Source: CAD feature listing. Evaluate the final solid. Frame: model axes, mm. A direction names the side the tool comes from. Give positions to 0.01 mm unless a question says otherwise; leave off trailing zeros. Order: outer loops, then holes, each group sorted by start corner. A loop starts at its lowest first (then second) coordinate and runs counter-clockwise, first axis right, second up.
```python
from build123d import *

# Parameters (mm, degrees)
SKETCH_1_W               = 994
SKETCH_1_H               = 740
EXTRUDE_1_DEPTH          = 4
CUT_EXTRUDE_3_DEPTH      = 1240.214267187
SKETCH_10_W              = 20
SKETCH_10_H              = 20
SKETCH_10_W_2            = 40
SKETCH_10_H_2            = 40
SKETCH_10_W_3            = 30
SKETCH_10_H_3            = 30
CUT_EXTRUDE_4_DEPTH      = 1240.214267187
SKETCH_11_W              = 11
SKETCH_11_H              = 15.8
CUT_EXTRUDE_5_DEPTH      = 1240.214267187
SKETCH_2_R               = 2.6
CUT_EXTRUDE_1_DEPTH      = 1240.214267187
SKETCH_12_W              = 8
SKETCH_12_H              = 20
CUT_EXTRUDE_6_DEPTH      = 1240.214267187
CUT_EXTRUDE_7_DEPTH      = 1240.214267187
CUT_EXTRUDE_7_DEPTH_BACK = 1240.214267187
SKETCH_13_W              = 4.2
SKETCH_13_H              = 20.2
SKETCH_6_W               = 26.45
SKETCH_6_H               = 740
EXTRUDE_2_DEPTH          = 4
SKETCH_8_W               = 5.8
SKETCH_8_H               = 10.5
CUT_EXTRUDE_2_DEPTH      = 1243.700125734
SKETCH_14_R              = 2.6
CUT_EXTRUDE_8_DEPTH      = 1243.700125734
FILLET_1_R               = 1.5
FILLET_2_R               = 5.5
FILLET_4_R               = 2.5


with BuildPart() as part:
    # Эскиз1 → Бобышка-Вытянуть1 (new body)
    with BuildSketch(Plane.XY):
        with Locations((497, 370)):
            Rectangle(SKETCH_1_W, SKETCH_1_H)
    extrude(amount=EXTRUDE_1_DEPTH)

    # Эскиз9 → Вырез-Вытянуть3 (cut, through all)
    with BuildSketch(Plane(origin=(0, 0, 0), x_dir=(-1, 0, 0), z_dir=(0, 0, -1))):
        Polygon((-689.6, -0.4), (-788.9, -0.4), (-788.9, 70.5), (-770.4, 70.5), (-770.4, 86.4), (-729.817747803, 86.4), (-689.6, 40.149590026), align=None)
        Polygon((-689.6, 740.4), (-802.9, 740.4), (-802.9, 669.5), (-770.4, 669.5), (-770.4, 653.6), (-729.817747803, 653.6), (-689.6, 699.850409974), align=None)
    extrude(amount=-CUT_EXTRUDE_3_DEPTH, mode=Mode.SUBTRACT)

    # Эскиз10 → Вырез-Вытянуть4 (cut, through all)
    with BuildSketch(Plane(origin=(0, 0, 0), x_dir=(-1, 0, 0), z_dir=(0, 0, -1))):
        with Locations((-692.63780609, 80.345862825)):
            Rectangle(SKETCH_10_W, SKETCH_10_H)
        with Locations((-904, 370)):
            Rectangle(SKETCH_10_W_2, SKETCH_10_H_2)
        with Locations((-692.63780609, 659.654137175)):
            Rectangle(SKETCH_10_W, SKETCH_10_H)
        with Locations((-715, 370)):
            Rectangle(SKETCH_10_W_3, SKETCH_10_H_3)
    extrude(amount=-CUT_EXTRUDE_4_DEPTH, mode=Mode.SUBTRACT)

    # Эскиз11 → Вырез-Вытянуть5 (cut, through all)
    with BuildSketch(Plane(origin=(0, 0, 0), x_dir=(-1, 0, 0), z_dir=(0, 0, -1))):
        with Locations((-798.5, 37.1)):
            Rectangle(SKETCH_11_W, SKETCH_11_H)
        with Locations((-812.5, 702.9)):
            Rectangle(SKETCH_11_W, SKETCH_11_H)
    extrude(amount=-CUT_EXTRUDE_5_DEPTH, mode=Mode.SUBTRACT)

    # Эскиз2 → Вырез-Вытянуть1 (cut, through all)
    with BuildSketch(Plane(origin=(0, 0, 0), x_dir=(-1, 0, 0), z_dir=(0, 0, -1))):
        with Locations((-10, 10)):
            Circle(SKETCH_2_R)
        with Locations((-10, 250)):
            Circle(SKETCH_2_R)
        with Locations((-10, 490)):
            Circle(SKETCH_2_R)
        with Locations((-10, 730)):
            Circle(SKETCH_2_R)
        with Locations((-984, 10)):
            Circle(SKETCH_2_R)
        with Locations((-984, 250)):
            Circle(SKETCH_2_R)
        with Locations((-984, 490)):
            Circle(SKETCH_2_R)
        with Locations((-984, 730)):
            Circle(SKETCH_2_R)
        with Locations((-233.33, 10)):
            Circle(SKETCH_2_R)
        with Locations((-233.33, 730)):
            Circle(SKETCH_2_R)
        with Locations((-456.66, 10)):
            Circle(SKETCH_2_R)
        with Locations((-456.66, 730)):
            Circle(SKETCH_2_R)
        with Locations((-679.99, 10)):
            Circle(SKETCH_2_R)
        with Locations((-679.99, 730)):
            Circle(SKETCH_2_R)
        with Locations((-799, 10)):
            Circle(SKETCH_2_R)
        with Locations((-814, 730)):
            Circle(SKETCH_2_R)
    extrude(amount=-CUT_EXTRUDE_1_DEPTH, mode=Mode.SUBTRACT)

    # Эскиз12 → Вырез-Вытянуть6 (cut, through all)
    with BuildSketch(Plane(origin=(0, 0, 0), x_dir=(-1, 0, 0), z_dir=(0, 0, -1))):
        with Locations((-760, 314)):
            Rectangle(SKETCH_12_W, SKETCH_12_H)
        with Locations((-740, 314)):
            Rectangle(SKETCH_12_W, SKETCH_12_H)
        with Locations((-760, 267)):
            Rectangle(SKETCH_12_W, SKETCH_12_H)
        with Locations((-760, 155)):
            Rectangle(SKETCH_12_W, SKETCH_12_H)
        with Locations((-760, 426)):
            Rectangle(SKETCH_12_W, SKETCH_12_H)
        with Locations((-760, 473)):
            Rectangle(SKETCH_12_W, SKETCH_12_H)
        with Locations((-760, 585)):
            Rectangle(SKETCH_12_W, SKETCH_12_H)
        with Locations((-740, 164)):
            Rectangle(SKETCH_12_W, SKETCH_12_H)
        with Locations((-740, 428)):
            Rectangle(SKETCH_12_W, SKETCH_12_H)
        with Locations((-740, 525.85)):
            Rectangle(SKETCH_12_W, SKETCH_12_H)
    extrude(amount=-CUT_EXTRUDE_6_DEPTH, mode=Mode.SUBTRACT)

    # Эскиз13 → Вырез-Вытянуть7 (cut, two sides: drawn at the far end of the back side and taken through both)
    with BuildSketch(Plane(origin=(0, 0, 0), x_dir=(-1, 0, 0), z_dir=(0, 0, -1)).offset(-CUT_EXTRUDE_7_DEPTH_BACK)):
        with Locations((-611.5, 20)):
            Rectangle(SKETCH_13_W, SKETCH_13_H)
        with Locations((-926, 20)):
            Rectangle(SKETCH_13_W, SKETCH_13_H)
        with Locations((-611.5, 160)):
            Rectangle(SKETCH_13_W, SKETCH_13_H)
        with Locations((-611.5, 300)):
            Rectangle(SKETCH_13_W, SKETCH_13_H)
        with Locations((-611.5, 440)):
            Rectangle(SKETCH_13_W, SKETCH_13_H)
        with Locations((-611.5, 580)):
            Rectangle(SKETCH_13_W, SKETCH_13_H)
        with Locations((-611.5, 720)):
            Rectangle(SKETCH_13_W, SKETCH_13_H)
        with Locations((-926, 160)):
            Rectangle(SKETCH_13_W, SKETCH_13_H)
        with Locations((-926, 300)):
            Rectangle(SKETCH_13_W, SKETCH_13_H)
        with Locations((-926, 440)):
            Rectangle(SKETCH_13_W, SKETCH_13_H)
        with Locations((-926, 580)):
            Rectangle(SKETCH_13_W, SKETCH_13_H)
        with Locations((-926, 720)):
            Rectangle(SKETCH_13_W, SKETCH_13_H)
    extrude(amount=CUT_EXTRUDE_7_DEPTH + CUT_EXTRUDE_7_DEPTH_BACK, mode=Mode.SUBTRACT)

    # Эскиз6 → Бобышка-Вытянуть2 (add)
    with BuildSketch(Plane(origin=(994, 0, 0), x_dir=(0, 0, -1), z_dir=(1, 0, 0))):
        with Locations((-13.225, 370)):
            Rectangle(SKETCH_6_W, SKETCH_6_H)
    extrude(amount=EXTRUDE_2_DEPTH)

    # Эскиз8 → Вырез-Вытянуть2 (cut, through all)
    with BuildSketch(Plane(origin=(998, 0, 0), x_dir=(0, 0, -1), z_dir=(1, 0, 0))):
        with Locations((-13.98, 145.25)):
            Rectangle(SKETCH_8_W, SKETCH_8_H)
        with Locations((-13.98, 162.25)):
            Rectangle(SKETCH_8_W, SKETCH_8_H)
        with Locations((-13.98, 577.75)):
            Rectangle(SKETCH_8_W, SKETCH_8_H)
        with Locations((-13.98, 594.75)):
            Rectangle(SKETCH_8_W, SKETCH_8_H)
    extrude(amount=-CUT_EXTRUDE_2_DEPTH, mode=Mode.SUBTRACT)

    # Эскиз14 → Вырез-Вытянуть8 (cut, through all)
    with BuildSketch(Plane(origin=(998, 0, 0), x_dir=(0, 0, -1), z_dir=(1, 0, 0))):
        with Locations((-14, 10)):
            Circle(SKETCH_14_R)
        with Locations((-14, 298)):
            Circle(SKETCH_14_R)
        with Locations((-14, 442)):
            Circle(SKETCH_14_R)
        with Locations((-14, 730)):
            Circle(SKETCH_14_R)
    extrude(amount=-CUT_EXTRUDE_8_DEPTH, mode=Mode.SUBTRACT)

    # Скругление1
    fillet_1_edges = [part.edges().sort_by_distance(p)[0] for p in [
        (994, 370, 4),
    ]]
    fillet(fillet_1_edges, radius=FILLET_1_R)

    # Скругление2
    fillet_2_edges = [part.edges().sort_by_distance(p)[0] for p in [
        (998, 370, 0),
    ]]
    fillet(fillet_2_edges, radius=FILLET_2_R)

    # Скругление4
    fillet_4_edges = [part.edges().sort_by_distance(p)[0] for p in [
        (689.6, 40.149590026, 2),
        (770.4, 70.5, 2),
        (770.4, 86.4, 2),
        (729.817747803, 86.4, 2),
        (689.6, 699.850409974, 2),
        (729.817747803, 653.6, 2),
        (770.4, 653.6, 2),
        (770.4, 669.5, 2),
    ]]
    fillet(fillet_4_edges, radius=FILLET_4_R)


solid = part.part
```
1) Reachability of faces 4 (the flat face through (709.914, 676.489, 1.972)), 5 (the flat face through (998, 375, 16)) from +Z, -Z, +X, -X, +Y, -Y: full face, straight path, thin tool, end or side. Return the list, or none.
Report:
face 4: +Z, -Z, +Y
face 5: +Z, -Z, +X, +Y, -Y
2) Material intervals for L1, parallel to Y at x = 799, z = 2.75; L2, parallel to Y at x = 984, z = 3.15; L3, parallel to X at y = 94, z = 13.25, sorted ascending.
Report:
L1: y = 0 to 7.4, 12.6 to 29.2, 45 to 669.5
L2: y = 0 to 7.4, 12.6 to 247.4, 252.6 to 487.4, 492.6 to 727.4, 732.6 to 740
L3: x = 994 to 998
3) Section query B-B, the plane y = 366.5. Return the cut outline in (x, z).
Report:
outline: (0, 0) - (700, 0) - (700, 4) - (0, 4) - close; (730, 0) - (884, 0) - (884, 4) - (730, 4) - close; (924, 0) - (992.5, 0) arc R5.5 ccw to (998, 5.5) - (998, 26.45) - (994, 26.45) - (994, 5.5) arc R1.5 cw to (992.5, 4) - (924, 4) - close
4) Draft query along X for faces 1 (the flat face through (994, 375, 16)), 2 (the flat face through (489, 375, 4)), 3 (the flat face through (709.914, 63.511, 1.972)). Return one class per face: +X half, -X half, draft (parallel to the pull), parting line (faces both ways), or undercut.
Report:
face 1: -X half
face 2: draft
face 3: undercut
5) Pin query (flat end, axial travel): pin 1 (3 mm diameter, centred on y = 317.5, z = 2.5, fed in from +X); pin 2 (1.2 mm diameter, centred on x = 761.5, z = 3, fed in from -Y); pin 3 (4 mm diameter, centred on y = 471.5, z = 22, fed in from -X); pin 4 (4 mm diameter, centred on x = 276.5, z = 7.5, fed in from +Y) (1 decimal). Return the tip coordinate at first contact, or that it passes through.
Report:
pin 1: stops at x = 997.79
pin 2: stops at y = 86.4
pin 3: stops at x = 994
pin 4: passes through
6) Section query A-A, the plane x = 904. Return the cut outline in (y, z).
Report:
outline: (0, 0) - (350, 0) - (350, 4) - (0, 4) - close; (390, 0) - (740, 0) - (740, 4) - (390, 4) - close
7) Section query D-D, the plane x = 664.5. Return the cut outline in (y, z).
Report:
outline: (0, 0) - (740, 0) - (740, 4) - (0, 4) - close
8) Section query C-C, the plane y = 558.5. Return the cut outline in (x, z), and give its area (3 significant figures).
Report:
outline: (0, 0) - (992.5, 0) arc R5.5 ccw to (998, 5.5) - (998, 26.45) - (994, 26.45) - (994, 5.5) arc R1.5 cw to (992.5, 4) - (0, 4) - close
area: 4,080 mm2
